from build123d import *

# Parameters (mm, degrees)
SKETCH1_W           = 152.4
SKETCH1_H           = 152.4
BOSS_EXTRUDE1_DEPTH = 8.466666667
SKETCH2_R           = 5.08
CUT_EXTRUDE1_DEPTH  = 6.35
BOSS_EXTRUDE3_DEPTH = 12.7
SKETCH4_R           = 21.697410495
CUT_EXTRUDE2_DEPTH  = 12.7


with BuildPart() as part:
    # Sketch1 → Boss-Extrude1 (new body)
    with BuildSketch(Plane(origin=(0, 0, 0), x_dir=(1, 0, 0), z_dir=(0, 1, 0))):
        Rectangle(SKETCH1_W, SKETCH1_H)
    extrude(amount=BOSS_EXTRUDE1_DEPTH)

    # Sketch2 → Cut-Extrude1 (cut)
    with BuildSketch(Plane(origin=(0, 0, 0), x_dir=(-1, 0, 0), z_dir=(0, -1, 0))):
        with Locations(Location((61.345958621, 44.67327441, 0), (0, 0, 90))):
            Circle(SKETCH2_R)
        with Locations(Location((0, -61.127341862, 0), (0, 0, 90))):
            Circle(SKETCH2_R)
        with Locations(Location((-61.729425139, 44.45, 0), (0, 0, 90))):
            Circle(SKETCH2_R)
    extrude(amount=-CUT_EXTRUDE1_DEPTH, mode=Mode.SUBTRACT)

    # Sketch3 → Boss-Extrude3 (add)
    with BuildSketch(Plane(origin=(0, 8.466666667, 0), x_dir=(1, 0, 0), z_dir=(0, 1, 0))):
        with BuildLine():
            Line((-52.940598994, -13.15996673), (-52.940598994, -67.121640926))
            Line((-52.940598994, -67.121640926), (52.940598994, -67.121640926))
            Line((52.940598994, -67.121640926), (52.940598994, -13.15996673))
            ThreePointArc((52.940598994, -13.15996673), (0, 69.962044891), (-52.940598994, -13.15996673))
        make_face()
        with BuildLine():
            Line((-46.590598994, -11.708782736), (-46.590598994, -60.771640926))
            Line((-46.590598994, -60.771640926), (46.590598994, -60.771640926))
            Line((46.590598994, -60.771640926), (46.590598994, -11.708782736))
            ThreePointArc((46.590598994, -11.708782736), (0, 63.612044891), (-46.590598994, -11.708782736))
        make_face(mode=Mode.SUBTRACT)
    extrude(amount=BOSS_EXTRUDE3_DEPTH)

    # Sketch4 → Cut-Extrude2 (cut)
    with BuildSketch(Plane(origin=(0, 8.466666667, 0), x_dir=(1, 0, 0), z_dir=(0, 1, 0))):
        with Locations(Location((0, -17.813493045, 0), (0, 0, 270))):
            Circle(SKETCH4_R)
    extrude(amount=-CUT_EXTRUDE2_DEPTH, mode=Mode.SUBTRACT)


solid = part.part
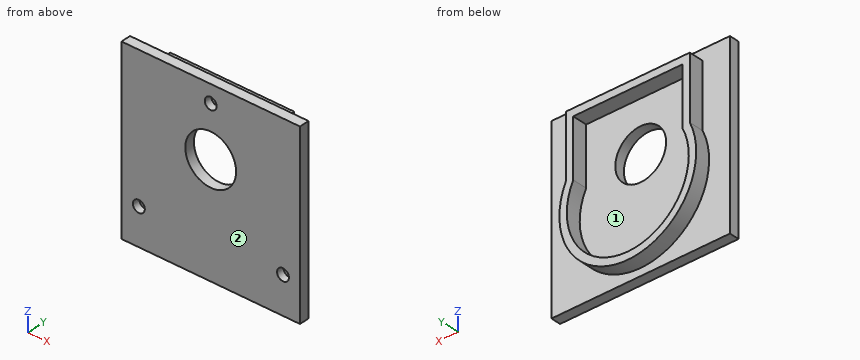
Read the model definition and answer for the solid it produces. Units are mm, in the model's axes. Face numbers are marked on the shaded views. Coordinates: 2 decimals unless noted, no trailing zeros. Write each loop counter-clockwise with the first axis right and the second up, starting at its lowest first coordinate (ties: lowest second). Pieces come first, ordered by that corner, then holes. Notation, with made-up numbers: M 54.25,-2.5 L 73.25,-2.5 A27 ccw 73.25,18.5 Z; hole C 64,80 d3. An arc over 180 degrees is marked long. Use a Markdown table: item, result.
Q1. The part is cut by section C-C, the plane y = 11. Write down the section's boundary in (x, z), then the cut area to 3 significant figures.
Answer block:
| item | result |
|---|---|
| outline | M -52.94,13.16 A58.42 ccw long 52.94,13.16 L 52.94,67.12 L -52.94,67.12 Z; hole M -46.59,11.71 A52.07 ccw long 46.59,11.71 L 46.59,60.77 L -46.59,60.77 Z |
| area | 2,700 mm2 |
Q2. The part is cut by section A-A, the plane x = 0. Write down the section's boundary in (y, z).
Answer block:
| item | result |
|---|---|
| outline | M 0,-76.2 L 8.47,-76.2 L 8.47,-69.96 L 21.17,-69.96 L 21.17,-63.61 L 8.47,-63.61 L 8.47,-3.88 L 0,-3.88 Z; M 0,39.51 L 8.47,39.51 L 8.47,60.77 L 21.17,60.77 L 21.17,67.12 L 8.47,67.12 L 8.47,76.2 L 0,76.2 L 0,66.21 L 6.35,66.21 L 6.35,56.05 L 0,56.05 Z |
Q3. Straight lines are drawn through the part: L1, parallel to X at y = 4.5, z = -44.45; L2, parallel to X at y = 12.25, z = 42.5; L3, parallel to Z at x = 1, y = 17.75. For each, find the intervals that lie inside material, in ascending order. Write a range as [from, to].
Answer block:
| item | result |
|---|---|
| L1 | x = [-76.2, -66.42], [-56.27, 56.65], [66.81, 76.2] |
| L2 | x = [-52.94, -46.59], [46.59, 52.94] |
| L3 | z = [-69.95, -63.6], [60.77, 67.12] |
Q4. Determine the mould class of the marked faces 1 and 2 for opening direction X: released by +X, released by -X, zero draft, split by the parting line, or undercut.
Answer block:
| item | result |
|---|---|
| face 1 | undercut |
| face 2 | zero draft |
Q5. The part is cut by section B-B, the plane z = 52.5. Write down the section's boundary in (x, y), then the cut area to 3 significant figures.
Answer block:
| item | result |
|---|---|
| outline | M -76.2,0 L 76.2,0 L 76.2,8.47 L 52.94,8.47 L 52.94,21.17 L 46.59,21.17 L 46.59,8.47 L -46.59,8.47 L -46.59,21.17 L -52.94,21.17 L -52.94,8.47 L -76.2,8.47 Z |
| area | 1,450 mm2 |
Q6. The part is cut by section D-D, the plane z = 30. Write down the section's boundary in (x, y).
Answer block:
| item | result |
|---|---|
| outline | M -76.2,0 L -17.95,0 L -17.95,8.47 L -46.59,8.47 L -46.59,21.17 L -52.94,21.17 L -52.94,8.47 L -76.2,8.47 Z; M 17.95,0 L 76.2,0 L 76.2,8.47 L 52.94,8.47 L 52.94,21.17 L 46.59,21.17 L 46.59,8.47 L 17.95,8.47 Z |
Q7. Each of these flat-tipped pins is pushed along its axis until it touches: pin 1 Ø10 at (y, z) = (17, 51.5) entering from +X; pin 2 Ø3 at (y, z) = (12.5, -53.5) entering from -X; pin 3 Ø1.5 at (x, z) = (-36, -27) entering from +Y. Where does it stop, or does it pass through?
Answer block:
| item | result |
|---|---|
| pin 1 | stops at x = 52.94 |
| pin 2 | stops at x = -42.14 |
| pin 3 | stops at y = 8.47 |
